Read the model definition and answer for the solid it produces. Units are mm, in the model's axes. Give positions to 0.01 mm unless a question says otherwise; leave off trailing zeros. Order: outer loops, then holes, each group sorted by start corner. A loop starts at its lowest first (then second) coordinate and runs counter-clockwise, first axis right, second up. Notation, with made-up numbers: M 63,-27.75 L 72,-27.75 A20 cw 72,5.25 Z; hole C 55,20 d1. An arc over 180 degrees is marked long. One line per item, written item: value. Start each with the question number.
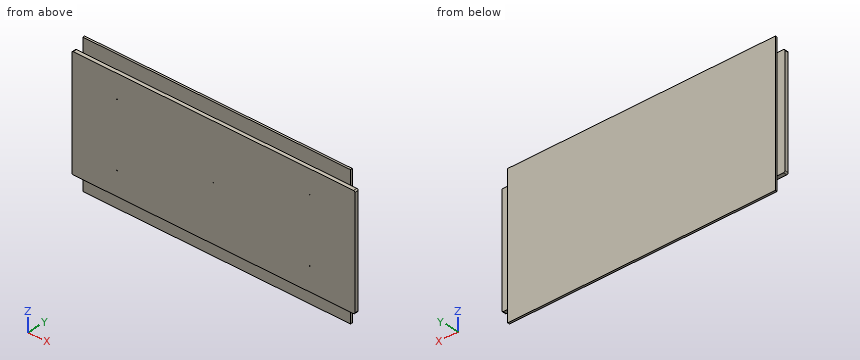
from build123d import *

# Parameters (mm, degrees)
SKETCH1_W                    = 1343.025
SKETCH1_H                    = 527.05
BOSS_EXTRUDE1_DEPTH          = 17.78
FILLET1_R                    = 6.35
F_1_8_0_125_DIAMETER_HOLE1_D = 3.175
SKETCH2_W                    = 1270
SKETCH2_H                    = 660.4
BOSS_EXTRUDE2_DEPTH          = 9.525


with BuildPart() as part:
    # Sketch1 → Boss-Extrude1 (new body)
    with BuildSketch(Plane(origin=(0, 0, 0), x_dir=(1, 0, 0), z_dir=(0, 1, 0))):
        Rectangle(SKETCH1_W, SKETCH1_H)
    extrude(amount=BOSS_EXTRUDE1_DEPTH)

    # Fillet1
    fillet1_edges = [part.edges().sort_by_distance(p)[0] for p in [
        (671.5125, 8.89, 263.525),
        (-671.5125, 8.89, 263.525),
        (-671.5125, 8.89, -263.525),
        (671.5125, 8.89, -263.525),
    ]]
    fillet(fillet1_edges, radius=FILLET1_R)

    # 1/8 (0.125) Diameter Hole1 (through all)
    with Locations(Plane(origin=(0, 17.78, 0), x_dir=(1, 0, 0), z_dir=(0, 1, 0))):
        with Locations((0, 0), (457.2, 152.4), (-457.2, -152.4), (-457.2, 152.4), (457.2, -152.4)):
            Hole(F_1_8_0_125_DIAMETER_HOLE1_D / 2)

    # Sketch2 → Boss-Extrude2 (add)
    with BuildSketch(Plane(origin=(0, 17.78, 0), x_dir=(1, 0, 0), z_dir=(0, 1, 0))):
        Rectangle(SKETCH2_W, SKETCH2_H)
    extrude(amount=BOSS_EXTRUDE2_DEPTH)


solid = part.part
Q1. Each of these flat-tipped pins is pushed along its axis until it touches: pin 1 (5 mm diameter, centred on x = 0, z = 0, fed in from -Y); pin 2 (3 mm diameter, centred on x = -194, y = 3, fed in from -Z) (3 decimals); pin 3 (5 mm diameter, centred on y = 24.5, z = 68.5, fed in from -X); pin 4 (1 mm diameter, centred on x = 0.5, z = -0.5, fed in from -Y). Where does it stop, or does it pass through?
Q2. Find section A-A, the plane y = 11.5. State how many separate pieces and enclosed holes the cut face has, then the cut area to 3 significant figures.
Q3. Find section B-B, the plane x = -403. Give the vertices of the cut face in (y, z) (3 decimals).
Q4. Consider probe 1 along X at (y, z) = (11.5, 152.4); probe 2 along Z at (x, y) = (-457.2, 7.5) (1 decimal); probe 3 along X at (y, z) = (18.75, 71). Determine where each line is inside the solid, lowest interval first.
Q5. Find section C-C, the plane z = -189. Give the vertices of the cut face in (x, y) (1 decimal).
Evaluation:
1. pin 1: y = 0
1. pin 2: z = -263.525
1. pin 3: x = -635
1. pin 4: y = 17.78
2. separate pieces: 1
2. enclosed holes: 5
2. area: 708,000 mm2
3. outline: M 0,-263.525 L 17.78,-263.525 L 17.78,-330.2 L 27.305,-330.2 L 27.305,330.2 L 17.78,330.2 L 17.78,263.525 L 0,263.525 Z
4. probe 1: -671.51 to -458.79, -455.61 to 455.61, 458.79 to 671.51
4. probe 2: -263.5 to -154, -150.8 to 150.8, 154 to 263.5
4. probe 3: -635 to 635
5. outline: M -671.5,0 L 671.5,0 L 671.5,17.8 L 635,17.8 L 635,27.3 L -635,27.3 L -635,17.8 L -671.5,17.8 Z
